Can you work these out from the model? Positions are in its coordinate system, mm. Round coordinates to 2 decimals unless told otherwise and drop trailing zeros. Loops run counter-clockwise (first coordinate to the right, second up) from the corner with the lowest first, then second, coordinate; pieces in that order, holes last. Notation, with made-up numbers: M 41.5,33.5 L 87.5,33.5 A18 ccw 87.5,67.5 Z; hole C 78.5,-13 d11. An arc over 180 degrees is marked long. Answer as CSV lines item,"result".
Autodesk Inventor part; units mm, degrees
ref_plane "YZ Plane" through (0, 0, 0) normal (1, 0, 0) x (0, 1, 0)
ref_plane "XZ Plane" through (0, 0, 0) normal (0, 1, 0) x (-1, 0, 0)
ref_plane "XY Plane" through (0, 0, 0) normal (0, 0, 1) x (1, 0, 0)
sketch "Skizze1" plane through (0, 0, 0) normal (0, 0, 1) x (1, 0, 0)
  line L0 (40, 180) -> (-40, 180)
  line L1 (-40, 180) -> (-40, -180)
  line L2 (-40, -180) -> (40, -180)
  line L3 (40, -180) -> (40, 180)
  line L4 (40, 180) -> (-40, -180) construction
  line L5 (-40, 180) -> (40, -180) construction
  point P0 (0, 0)
  dimension "d0" = 80
  dimension "d1" = 360
extrude "Extrusion1" add sketch "Skizze1" along normal blind 10
sketch "Skizze2" plane through (0, 0, 10) normal (0, 0, 1) x (1, 0, 0)
  line L0 (40, 180) -> (-40, 180)
  line L1 (40, -180) -> (40, 180)
  point P0 (0, 0)
  point P1 (25, 110)
  dimension "d16" = 15
  dimension "d17" = 70
hole "Bohrung2" at (25, 110, 10) direction (0, 0, -1) diameter 6 end through all
sketch "Skizze3" plane through (0, 0, 0) normal (0, 0, -1) x (-1, 0, 0)
  circle A0 centre (-25, 110) radius 3
  line L0 (40, 180) -> (40, -180)
  line L1 (-25, 92.5) -> (-25, 127.5) construction
  point P0 (0, 0)
  dimension "d25" = 35
hole "Bohrung3" at (25, 92.5, 0) at (25, 127.5, 0) direction (0, 0, 1) diameter 4.5 end through all countersink diameter 10 countersink angle 90
sketch "Skizze4" plane through (0, 0, 10) normal (0, 0, 1) x (1, 0, 0)
  line L0 (-40, 180) -> (-40, -180)
  line L1 (-40, -180) -> (40, -180)
  line L2 (40, -180) -> (40, 180)
  line L3 (15, -135) -> (15, -150) construction
  point P0 (0, 0)
  dimension "d34" = 15
  dimension "d35" = 30
  dimension "d36" = 55
hole "Bohrung4" at (15, -150, 10) at (15, -135, 10) direction (0, 0, -1) diameter 3.242 end through all
pattern_linear "Rechteckige Anordnung2" count 2 spacing 200 along (0, 1, 0) of "Bohrung4"
sketch "Skizze5" plane through (-40, -180, 0) normal (0, -1, 0) x (1, 0, 0)
  line L0 (0, 0) -> (80, 0)
  line L1 (0, 0) -> (0, 10)
  line L2 (5, 5) -> (75, 5)
  point P0 (40, 0)
  point P1 (40, 5)
  point P2 (40, 0)
  point P3 (0, 5)
  dimension "d47" = 5
hole "Bohrung5" at (-35, -180, 5) at (35, -180, 5) direction (0, 1, 0) diameter 3.242 depth 10 tip angle 118
properties part number "Tunel_SidePanel" material "Polycarbonat, klar"
Item 1: If I drill on line 1 along Y through (x, z) = (15, 4); line 2 along Y through (x, z) = (25, 5); line 3 along X through (y, z) = (92.5, 6.5), over which ranges is the centre line in solid material (lowest first)? Write a range as from..to.
Output:
line 1,"y = -180..-151.62, -148.38..-136.62, -133.38..48.38, 51.62..63.38, 66.62..180"
line 2,"y = -180..90.25, 94.75..107, 113..125.25, 129.75..180"
line 3,"x = -40..22.75, 27.25..40"
Item 2: If we section it at A-A on y = 110: Write out the boundary of the cut face in (x, z), then the cut area to 3 significant figures.
Output:
outline,"M -40,0 L 22,0 L 22,10 L -40,10 Z; M 28,0 L 40,0 L 40,10 L 28,10 Z"
area,"740 mm2"
Item 3: Will these pins go through, and if not, where does the flat tip stop? pin 1 (1.9 mm diameter, centred on x = 15, y = 65, fed in from +Z); pin 2 (5 mm diameter, centred on x = 25, y = 92.5, fed in from -Z).
Output:
pin 1,"passes through"
pin 2,"stops at z = 2.5"
Item 4: We'd pull the mould along X, two halves only. Please class faces 1 (the face through (-1, 3, 0)), 2 (the face through (25.73, 129.81, 2.58)), 3 (the face through (40, -3, 5)): released by +X, released by -X, zero draft, split by the parting line, or undercut.
Output:
face 1,"zero draft"
face 2,"undercut"
face 3,"released by +X"
